Could you check a few things on this drawing? It's one solid part, dimensions in mm from its lowest x, y, z. A direction names the side the tool comes from. Coordinates: 2 decimals unless noted, no trailing zeros. Write each loop counter-clockwise with the first axis right and the second up, starting at its lowest first coordinate (ties: lowest second). Pieces come first, ordered by that corner, then holes. Notation, with made-up numbers: M -16.75,18.25 L 13.25,18.25 A29 cw 13.25,53.25 Z; hole C 27,78.5 d1. An arc over 180 degrees is marked long. Use a Markdown table: item, result.
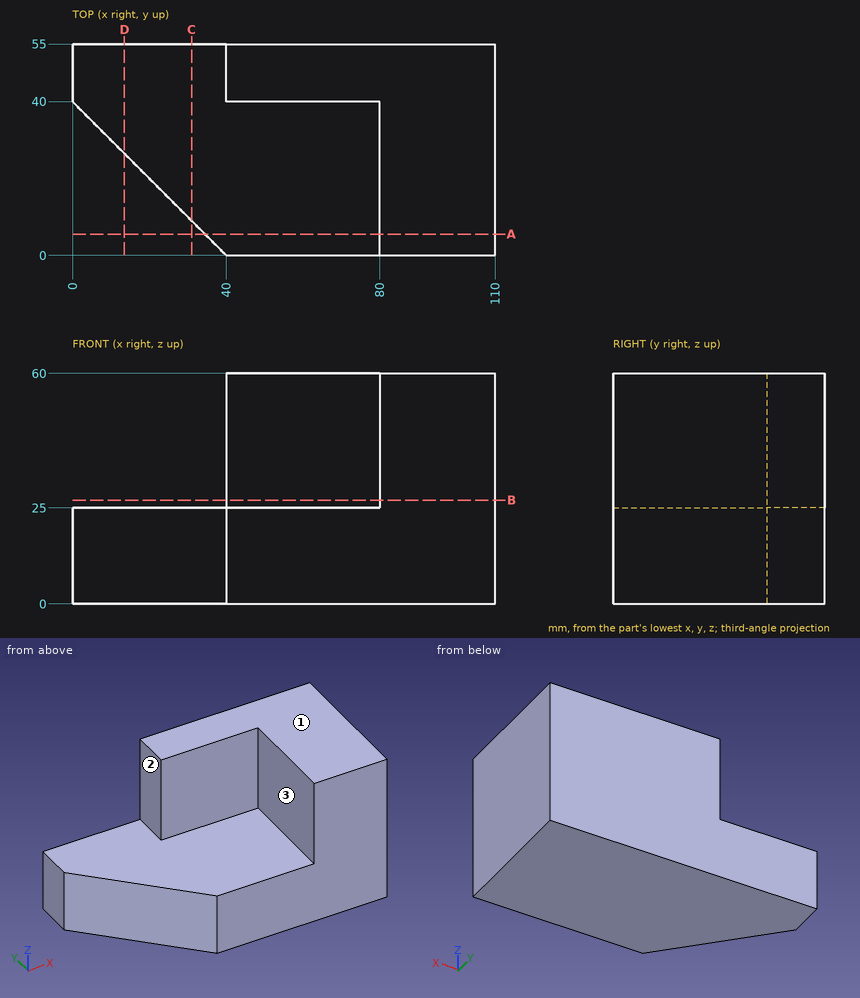
1. I need wall thicknesses on probe 1 along Z at (x, y) = (69.5, 11.5); probe 2 along Y at (x, z) = (40.5, 52.5); probe 3 along X at (y, z) = (36, 26.5). Which ranges of each line are inside material? Lowest first, please.
Answers follow:
| item | result |
|---|---|
| probe 1 | z = 0 to 25 |
| probe 2 | y = 40 to 55 |
| probe 3 | x = 80 to 110 |
2. Will these pins go through, and if not, where does the flat tip stop? pin 1 Ø17.5 at (x, z) = (51, 50.5) entering from -Y; pin 2 Ø2 at (y, z) = (6, 32.5) entering from -X; pin 3 Ø2 at (y, z) = (23, 12.5) entering from -X.
Answers follow:
| item | result |
|---|---|
| pin 1 | stops at y = 40 |
| pin 2 | stops at x = 80 |
| pin 3 | stops at x = 16 |
3. Suppose I cut it at A-A on y = 5.5. Write out the boundary of the cut face in (x, z), and give its area (3 significant figures).
Answers follow:
| item | result |
|---|---|
| outline | M 34.5,0 L 110,0 L 110,60 L 80,60 L 80,25 L 34.5,25 Z |
| area | 2,940 mm2 |
4. Suppose I cut it at B-B on z = 27. Write out the boundary of the cut face in (x, y), and give its area (3 significant figures).
Answers follow:
| item | result |
|---|---|
| outline | M 40,40 L 80,40 L 80,0 L 110,0 L 110,55 L 40,55 Z |
| area | 2,250 mm2 |
5. Suppose I cut it at D-D on x = 13.5. Write out the boundary of the cut face in (y, z).
Answers follow:
| item | result |
|---|---|
| outline | M 26.5,0 L 55,0 L 55,25 L 26.5,25 Z |
6. Suppose I cut it at C-C on x = 31. Write out the boundary of the cut face in (y, z).
Answers follow:
| item | result |
|---|---|
| outline | M 9,0 L 55,0 L 55,25 L 9,25 Z |
7. Which directions (+Z, -Z, +X, -X, +Y, -Y) give clear straight access to the entire face, cutting with the end or side of a thin tool? Please do the marked faces 1, 2 and 3.
Answers follow:
| item | result |
|---|---|
| face 1 | +Z, +X, -X, +Y, -Y |
| face 2 | +Z, -X, +Y, -Y |
| face 3 | +Z, -X, -Y |
